Can you work these out from the model? Positions are in its coordinate system, mm. Face numbers are marked on the shaded views. Give positions to 0.01 mm unless a question says otherwise; leave off trailing zeros. Write each loop counter-clockwise with the first axis right and the second up, starting at its lowest first coordinate (ties: lowest second). Pieces come first, ordered by that corner, then holes. Notation, with made-up numbers: (36, 65) -> (95, 65) arc R27 ccw to (95, 88) -> close; hole circle Ø7 at (-8.5, 72). An arc over 180 degrees is marked (long way). One line per item, written item: value.
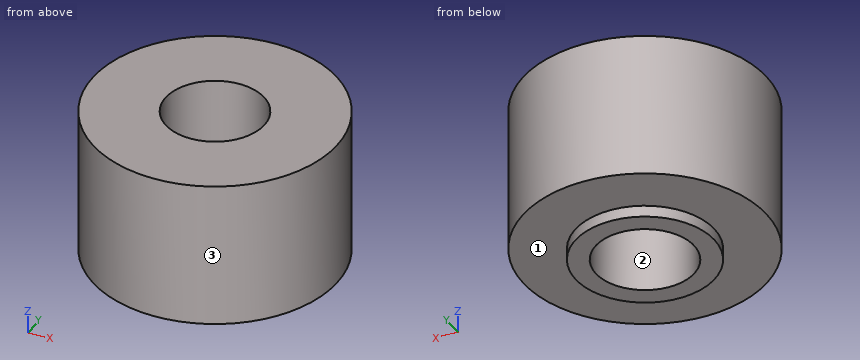
from build123d import *

# Parameters (mm, degrees)
SKETCH1_W           = 3.125
SKETCH1_H           = 3.75
SKETCH2_R           = 5.25
SKETCH2_R_2         = 2.125
BOSS_EXTRUDE1_DEPTH = 3.0725
SKETCH3_R           = 5.25
SKETCH3_R_2         = 3
CUT_EXTRUDE1_DEPTH  = 0.5


with BuildPart() as part:
    # Sketch1 → Revolve1 (revolve)
    with BuildSketch(Plane(origin=(0, 0, 0), x_dir=(1, 0, 0), z_dir=(0, 1, 0))):
        with Locations((3.6875, -1.875)):
            Rectangle(SKETCH1_W, SKETCH1_H)
    revolve(axis=Axis((0, 0, 0), (0, 0, 1)))

    # Sketch2 → Boss-Extrude1 (add)
    with BuildSketch(Plane.XY.offset(3.75)):
        Circle(SKETCH2_R)
        Circle(SKETCH2_R_2, mode=Mode.SUBTRACT)
    extrude(amount=BOSS_EXTRUDE1_DEPTH)

    # Sketch3 → Cut-Extrude1 (cut)
    with BuildSketch(Plane(origin=(0, 0, 0), x_dir=(-1, 0, 0), z_dir=(0, 0, -1))):
        Circle(SKETCH3_R)
        Circle(SKETCH3_R_2, mode=Mode.SUBTRACT)
    extrude(amount=-CUT_EXTRUDE1_DEPTH, mode=Mode.SUBTRACT)


solid = part.part
1) If we section it at D-D (y = -3.75): Write out the boundary of the cut face in (x, z), and give its area (3 significant figures).
Answer list:
outline: (-3.67, 0.5) -> (3.67, 0.5) -> (3.67, 6.82) -> (-3.67, 6.82) -> close
area: 46.5 mm^2
2) I need wall thicknesses on L1, parallel to Y at x = 0, z = 4 (3 decimals); L2, parallel to Z at x = -4.25, y = -2.25; L3, parallel to Y at x = 1.75, z = 1.5. Which ranges of each line are inside material? Lowest first, please.
Answer list:
L1: y = -5.25 to -2.125, 2.125 to 5.25
L2: z = 0.5 to 6.82
L3: y = -4.95 to -1.21, 1.21 to 4.95
3) If we section it at C-C (z = 5.75): Write out the boundary of the cut face in (x, y) (3 decimals).
Answer list:
outline: circle Ø10.5 at (0, 0); hole circle Ø4.25 at (0, 0)
4) Will these pins go through, and if not, where does the flat tip stop? pin 1 (2 mm diameter, centred on x = 3.5, z = 5, fed in from +Y); pin 2 (4 mm diameter, centred on y = 4, z = 4, fed in from -X).
Answer list:
pin 1: stops at y = 4.62
pin 2: stops at x = -4.85
5) We'd pull the mould along Y, two halves only. Please class the marked faces 1, 2 and 3: released by +Y, released by -Y, zero draft, split by the parting line, or undercut.
Answer list:
face 1: zero draft
face 2: undercut
face 3: split by the parting line
